Input: part model. Units: mm. Frame: model coordinates. Face numbers are marked on the shaded views. A direction names the side the tool comes from. Round coordinates to 2 decimals unless told otherwise and drop trailing zeros. Loops run counter-clockwise (first coordinate to the right, second up) from the corner with the lowest first, then second, coordinate; pieces in that order, holes last. Notation, with made-up numbers: (-32, -12) -> (0, -12) arc R26 ccw to (0, 22) -> close; hole circle Ø7 at (-32, 86.5). An arc over 180 degrees is marked (long way). Answer as a JSON object with one key per item and string values.
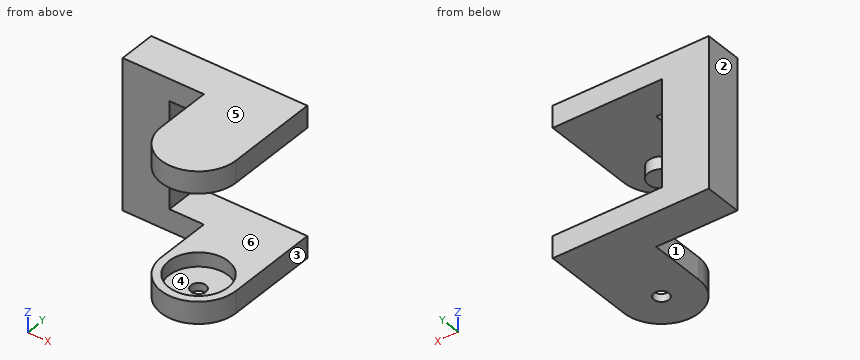
```python
from build123d import *

# Parameters (mm, degrees)
SKETCH1_R           = 9.5
BOSS_EXTRUDE1_DEPTH = 48
SKETCH2_W           = 34
SKETCH2_H           = 30
CUT_EXTRUDE1_DEPTH  = 62.481704596
BOSS_EXTRUDE2_START = -2.5
SKETCH3_R           = 9.5
SKETCH3_R_2         = 2.4
BOSS_EXTRUDE2_DEPTH = 2.5
SKETCH4_R           = 9.5
SKETCH4_R_2         = 4.2
BOSS_EXTRUDE3_DEPTH = 7
SKETCH5_R           = 4.2
BOSS_EXTRUDE4_DEPTH = 11
BOSS_EXTRUDE5_DEPTH = 48
SKETCH7_W           = 35
SKETCH7_H           = 34
CUT_EXTRUDE2_DEPTH  = 14.5


with BuildPart() as part:
    # Sketch1 → Boss-Extrude1 (new body)
    with BuildSketch(Plane.XY):
        with BuildLine():
            Line((-12, 0), (-12, 30))
            Line((-12, 30), (12, 30))
            Line((12, 30), (12, 0))
            ThreePointArc((12, 0), (0, -12), (-12, 0))
        make_face()
        Circle(SKETCH1_R, mode=Mode.SUBTRACT)
    extrude(amount=-BOSS_EXTRUDE1_DEPTH)

    # Sketch2 → Cut-Extrude1 (cut, through all)
    with BuildSketch(Plane.ZY.offset(12)):
        with Locations((-24, 3)):
            Rectangle(SKETCH2_W, SKETCH2_H)
    extrude(amount=-CUT_EXTRUDE1_DEPTH, mode=Mode.SUBTRACT)

    # Sketch3 → Boss-Extrude2 (add)
    with BuildSketch(Plane(origin=(0, 0, -48), x_dir=(-1, 0, 0), z_dir=(0, 0, -1)).offset(BOSS_EXTRUDE2_START)):
        Circle(SKETCH3_R)
        Circle(SKETCH3_R_2, mode=Mode.SUBTRACT)
    extrude(amount=BOSS_EXTRUDE2_DEPTH)

    # Sketch4 → Boss-Extrude3 (add)
    with BuildSketch(Plane.XY):
        with Locations(Location((0, 0, 0), (0, 0, 180))):
            Circle(SKETCH4_R)
        Circle(SKETCH4_R_2, mode=Mode.SUBTRACT)
    extrude(amount=-BOSS_EXTRUDE3_DEPTH)

    # Sketch5 → Boss-Extrude4 (add)
    with BuildSketch(Plane.XY):
        Circle(SKETCH5_R)
    extrude(amount=-BOSS_EXTRUDE4_DEPTH)

    # Sketch6 → Boss-Extrude5 (add)
    with BuildSketch(Plane(origin=(0, 0, -48), x_dir=(-1, 0, 0), z_dir=(0, 0, -1))):
        Polygon((12, 30), (12, 18), (18, 18), (38, 18), (38, 30), align=None)
    extrude(amount=-BOSS_EXTRUDE5_DEPTH)

    # Sketch7 → Cut-Extrude2 (cut)
    with BuildSketch(Plane(origin=(0, 30, 0), x_dir=(1, 0, 0), z_dir=(0, 1, 0))):
        with Locations((-5.5, 24)):
            Rectangle(SKETCH7_W, SKETCH7_H)
    extrude(amount=-CUT_EXTRUDE2_DEPTH, mode=Mode.SUBTRACT)


solid = part.part
```
1) Section C-C, the plane y = 24.5. Output: boundary loops of the cut face in (x, z), plus the area to 3 significant figures.
Output:
{"outline": "(-38, -48) -> (12, -48) -> (12, -41) -> (-23, -41) -> (-23, -7) -> (12, -7) -> (12, 0) -> (-38, 0) -> close", "area": "1,210 mm^2"}
2) Reachability of the marked faces 1 and 2 from +Z, -Z, +X, -X, +Y, -Y: full face, straight path, thin tool, end or side. Return the list, or none.
Output:
{"face 1": "+Z, -Z, -X, -Y", "face 2": "+Z, -Z, -X, +Y, -Y"}
3) Contact query for flat-ended pins moving along their axis: P1, Ø4.5, axis at x = 0, y = 0, coming from the -Z side; P2, Ø9.5, axis at y = 26, z = -17, coming from the +X side; P3, Ø13, axis at x = -23.5, z = -17.5, coming from the -Y side. Output: stop coordinate, or through.
Output:
{"P1": "stops at z = -11", "P2": "stops at x = -23", "P3": "stops at y = 18"}
4) Draft query along Z for the marked faces 3, 4, 5 and 6. Return one class per face: +Z half, -Z half, draft (parallel to the pull), parting line (faces both ways), or undercut.
Output:
{"face 3": "draft", "face 4": "undercut", "face 5": "+Z half", "face 6": "undercut"}
5) Section D-D, the plane x = -8.5. Output: boundary loops of the cut face in (y, z).
Output:
{"outline": "(-8.47, -48) -> (30, -48) -> (30, -41) -> (4.24, -41) -> (4.24, -45.5) -> (-4.24, -45.5) -> (-4.24, -41) -> (-8.47, -41) -> close; (-8.47, -7) -> (30, -7) -> (30, 0) -> (-8.47, 0) -> close"}
6) Section B-B, the plane x = -15.5. Output: boundary loops of the cut face in (y, z), plus the area to 3 significant figures.
Output:
{"outline": "(18, -48) -> (30, -48) -> (30, -41) -> (18, -41) -> close; (18, -7) -> (30, -7) -> (30, 0) -> (18, 0) -> close", "area": "168 mm^2"}
7) Section A-A, the plane x = 0. Output: boundary loops of the cut face in (y, z), plus the area to 3 significant figures.
Output:
{"outline": "(-12, -48) -> (-2.4, -48) -> (-2.4, -45.5) -> (-9.5, -45.5) -> (-9.5, -41) -> (-12, -41) -> close; (-12, -7) -> (-4.2, -7) -> (-4.2, -11) -> (4.2, -11) -> (4.2, -7) -> (30, -7) -> (30, 0) -> (-12, 0) -> close; (2.4, -48) -> (30, -48) -> (30, -41) -> (9.5, -41) -> (9.5, -45.5) -> (2.4, -45.5) -> close", "area": "524 mm^2"}
8) Ray query, probe 1 along Z at (x, y) = (-10.5, 24); probe 2 along Z at (x, y) = (-2.5, 2); probe 3 along Y at (x, z) = (0, -47.2). Return the intervals inside material, ascending.
Output:
{"probe 1": "z = -48 to -41, -7 to 0", "probe 2": "z = -48 to -45.5, -11 to 0", "probe 3": "y = -12 to -2.4, 2.4 to 30"}
